The listing builds one solid part. Answer for the finished solid, in the listing's coordinates (mm). A direction names the side the tool comes from. Give positions to 0.01 mm unless a question says otherwise; leave off trailing zeros. Order: outer loops, then holes, each group sorted by start corner. A loop starts at its lowest first (then second) coordinate and runs counter-clockwise, first axis right, second up. Notation, with made-up numbers: (87.25, 36) - (137.25, 36) arc R12 cw to (137.25, 59) - close; hole circle Ø8 at (86, 55.25). An arc over 180 degrees is marked (long way). Answer in a Markdown table with one row per item. Add a question column.
```python
from build123d import *

# Parameters (mm, degrees)
BOSS_EXTRUDE1_DEPTH = 6.35
SKETCH2_W           = 100
SKETCH2_H           = 93
BOSS_EXTRUDE2_DEPTH = 20
FILLET1_R           = 3.175
BOSS_EXTRUDE3_DEPTH = 31.5
SKETCH5_W           = 35.56
SKETCH5_H           = 35.56
CUT_EXTRUDE1_DEPTH  = 0.254
LPATTERN1_COUNT     = 3
LPATTERN1_PITCH     = 45.72
LPATTERN2_COUNT     = 2
LPATTERN2_PITCH     = 45.72


with BuildPart() as part:
    # Sketch1 → Boss-Extrude1 (new body)
    with BuildSketch(Plane(origin=(0, 0, 0), x_dir=(1, 0, 0), z_dir=(0, 1, 0))):
        with BuildLine():
            Line((-76.2, 95.25), (76.2, 95.25))
            ThreePointArc((76.2, 95.25), (85.725, 0), (76.2, -95.25))
            Line((76.2, -95.25), (-76.2, -95.25))
            ThreePointArc((-76.2, -95.25), (-85.725, 0), (-76.2, 95.25))
        make_face()
    extrude(amount=BOSS_EXTRUDE1_DEPTH)

    # Sketch2 → Boss-Extrude2 (add)
    with BuildSketch(Plane(origin=(0, 6.35, 0), x_dir=(1, 0, 0), z_dir=(0, 1, 0))):
        with Locations((0, 37.75)):
            Rectangle(SKETCH2_W, SKETCH2_H)
    extrude(amount=BOSS_EXTRUDE2_DEPTH)

    # Fillet1
    fillet1_edges = [part.edges().sort_by_distance(p)[0] for p in [
        (50, 16.35, 8.75),
        (50, 16.35, -84.25),
        (-50, 16.35, -84.25),
        (-50, 16.35, 8.75),
        (50, 26.35, -37.75),
        (0, 26.35, -84.25),
        (-50, 26.35, -37.75),
        (0, 26.35, 8.75),
    ]]
    fillet(fillet1_edges, radius=FILLET1_R)

    # Sketch3 → Boss-Extrude3 (add)
    with BuildSketch(Plane.XY.offset(8.75)):
        Polygon((-12, 6.35), (-12, 10.35), (-8, 10.35), (-8, 8.35), (-10, 8.35), (-10, 6.35), align=None)
        Polygon((10, 6.35), (12, 6.35), (12, 10.35), (8, 10.35), (8, 8.35), (10, 8.35), align=None)
    extrude(amount=BOSS_EXTRUDE3_DEPTH)

    # Sketch5 → Cut-Extrude1 (cut)
    with BuildSketch(Plane.XZ):
        with Locations((-45.72, -22.86)):
            Rectangle(SKETCH5_W, SKETCH5_H)
        with Locations((0, -22.86)):
            Rectangle(SKETCH5_W, SKETCH5_H)
        with Locations((45.72, -22.86)):
            Rectangle(SKETCH5_W, SKETCH5_H)
    cut_extrude1 = extrude(amount=-CUT_EXTRUDE1_DEPTH, mode=Mode.SUBTRACT)

    # LPattern1: Cut-Extrude1 ×3
    with Locations(*[(0, 0, i * LPATTERN1_PITCH) for i in range(1, LPATTERN1_COUNT)]):
        add(cut_extrude1, mode=Mode.SUBTRACT)

    # LPattern2: Cut-Extrude1 ×2
    with Locations(*[(0, 0, -i * LPATTERN2_PITCH) for i in range(1, LPATTERN2_COUNT)]):
        add(cut_extrude1, mode=Mode.SUBTRACT)


solid = part.part
```
(1) Find section D-D, the plane x = 1.5. Write down the section's boundary in (y, z) (3 decimals), plus the area to 3 significant figures.
(2) Find section B-B, the plane y = 17. Write down the section's boundary in (x, z) (3 decimals).
(3) Each of these flat-tipped pins is pushed along its axis until it touches: P1, Ø18, axis at x = 38.5, z = -15, coming from the -Y side; P2, Ø2, axis at x = -36, y = 21, coming from the -Z side; P3, Ø6, axis at y = 5, z = -49.5, coming from the -X side. Where does it stop, or does it pass through?
(4) The mould has two halves that part along X. Classify faces 1 (the face through (-85.723, 3.131, 1.342)), 2 (the face through (-46, 0.254, -68)), 3 (the face through (1, 3, 95.25)): +X half, -X half, draft (parallel to the pull), parting line (faces both ways), or undercut.
(5) Straight lines are drawn through the part: line 1 (X direction, y = 8, z = 18); line 2 (Z direction, x = 37, y = 7.5); line 3 (Y direction, x = -45, z = 21). For each, find the intervals that lie inside material, in ascending order.
(6) Find section A-A, the plane x = 53. Write down the section's boundary in (y, z), plus the area to 3 significant figures.
(7) Find section C-C, the plane z = -23. Write down the section's boundary in (x, y) (3 decimals), plus the area to 3 significant figures.
(8) For faces 4 (the face through (12, 8, 24)), 5 (the face through (1, 0, -1)), 6 (the face through (10, 10.35, 24)), 7 (the face through (-46, 0.254, -23)), determine the directions among +Z, -Z, +X, -X, +Y, -Y from which every point of the face is accessible in a straight line to the end or side of a thin tool.
Answer key:
| question | item | result |
|---|---|---|
| 1 | outline | (0, -95.25) - (6.35, -95.25) - (6.35, -84.25) - (23.175, -84.25) arc R3.175 ccw to (26.35, -81.075) - (26.35, 5.575) arc R3.175 ccw to (23.175, 8.75) - (6.35, 8.75) - (6.35, 95.25) - (0, 95.25) - (0, 86.36) - (0.254, 86.36) - (0.254, 50.8) - (0, 50.8) - (0, 40.64) - (0.254, 40.64) - (0.254, 5.08) - (0, 5.08) - (0, -5.08) - (0.254, -5.08) - (0.254, -40.64) - (0, -40.64) - (0, -50.8) - (0.254, -50.8) - (0.254, -86.36) - (0, -86.36) - close |
| 1 | area | 3,030 mm² |
| 2 | outline | (-50, -81.075) arc R3.175 ccw to (-46.825, -84.25) - (46.825, -84.25) arc R3.175 ccw to (50, -81.075) - (50, 5.575) arc R3.175 ccw to (46.825, 8.75) - (-46.825, 8.75) arc R3.175 ccw to (-50, 5.575) - close |
| 3 | P1 | y = 0.25 |
| 3 | P2 | z = -84.25 |
| 3 | P3 | x = -83.47 |
| 4 | face 1 | -X half |
| 4 | face 2 | undercut |
| 4 | face 3 | draft |
| 5 | line 1 | -12 to -10, 10 to 12 |
| 5 | line 2 | -84.25 to 8.75 |
| 5 | line 3 | 0.25 to 6.35 |
| 6 | outline | (0, -95.25) - (6.35, -95.25) - (6.35, 95.25) - (0, 95.25) - (0, 86.36) - (0.25, 86.36) - (0.25, 50.8) - (0, 50.8) - (0, 40.64) - (0.25, 40.64) - (0.25, 5.08) - (0, 5.08) - (0, -5.08) - (0.25, -5.08) - (0.25, -40.64) - (0, -40.64) - (0, -50.8) - (0.25, -50.8) - (0.25, -86.36) - (0, -86.36) - close |
| 6 | area | 1,170 mm² |
| 7 | outline | (-85.175, 0) - (-63.5, 0) - (-63.5, 0.254) - (-27.94, 0.254) - (-27.94, 0) - (-17.78, 0) - (-17.78, 0.254) - (17.78, 0.254) - (17.78, 0) - (27.94, 0) - (27.94, 0.254) - (63.5, 0.254) - (63.5, 0) - (85.175, 0) - (85.175, 6.35) - (50, 6.35) - (50, 23.175) arc R3.175 ccw to (46.825, 26.35) - (-46.825, 26.35) arc R3.175 ccw to (-50, 23.175) - (-50, 6.35) - (-85.175, 6.35) - close |
| 7 | area | 3,050 mm² |
| 8 | face 4 | +Z, +X, +Y |
| 8 | face 5 | +Z, -Z, +X, -X, -Y |
| 8 | face 6 | +Z, +X, -X, +Y |
| 8 | face 7 | -Y |
